The listing builds one solid part. Answer for the finished solid, in the listing's coordinates (mm). Coordinates: 2 decimals unless noted, no trailing zeros. Loops run counter-clockwise (first coordinate to the right, second up) from the corner with the lowest first, then second, coordinate; pieces in that order, holes last. Notation, with made-up numbers: (62.25, 19.25) - (69.25, 19.25) arc R31 cw to (69.25, 47.25) - close; hole circle Ø9 at (3.25, -14.5). An arc over 180 degrees is marked (long way). Put each result on its own line as item: value.
Autodesk Inventor part; units mm, degrees
ref_plane "YZ Plane" through (0, 0, 0) normal (1, 0, 0) x (0, 1, 0)
ref_plane "XZ Plane" through (0, 0, 0) normal (0, 1, 0) x (-1, 0, 0)
ref_plane "XY Plane" through (0, 0, 0) normal (0, 0, 1) x (1, 0, 0)
sketch "Эскиз1" plane through (0, 0, 0) normal (0, 0, 1) x (1, 0, 0)
  arc A0 (68.75, 375.75) -> (58.75, 375.75) centre (63.75, 375.75) ccw
  arc A1 (53.75, 266.5202) -> (58.75, 271.5202) centre (53.75, 271.5202) ccw
  arc A2 (58.75, 246.5202) -> (53.75, 251.5202) centre (53.75, 246.5202) ccw
  arc A3 (-312.25, 375.75) -> (-322.25, 375.75) centre (-317.25, 375.75) ccw
  arc A4 (-312.25, 271.5202) -> (-307.25, 266.5202) centre (-307.25, 271.5202) ccw
  arc A5 (-307.25, 251.5202) -> (-312.25, 246.5202) centre (-307.25, 246.5202) ccw
  arc A6 (-322.25, -155.2817) -> (-312.25, -155.2817) centre (-317.25, -155.2817) ccw
  arc A7 (58.75, -155.2817) -> (68.75, -155.2817) centre (63.75, -155.2817) ccw
  line L0 (68.75, -155.2817) -> (68.75, 375.75)
  line L1 (58.75, 375.75) -> (58.75, 271.5202)
  line L2 (53.75, 266.5202) -> (-307.25, 266.5202)
  line L3 (-307.25, 251.5202) -> (53.75, 251.5202)
  line L4 (58.75, 246.5202) -> (58.75, -155.2817)
  line L5 (-312.25, -155.2817) -> (-312.25, 246.5202)
  line L6 (-312.25, 271.5202) -> (-312.25, 375.75)
  line L7 (-322.25, 375.75) -> (-322.25, -155.2817)
  line L8 (-307.25, 267.0202) -> (53.75, 267.0202)
  arc A8 (53.75, 267.0202) -> (58.25, 271.5202) centre (53.75, 271.5202) ccw
  line L9 (58.25, 271.5202) -> (58.25, 375.75)
  arc A9 (69.25, 375.75) -> (58.25, 375.75) centre (63.75, 375.75) ccw
  line L10 (69.25, 375.75) -> (69.25, -155.2817)
  arc A10 (58.25, -155.2817) -> (69.25, -155.2817) centre (63.75, -155.2817) ccw
  line L11 (58.25, -155.2817) -> (58.25, 246.5202)
  arc A11 (58.25, 246.5202) -> (53.75, 251.0202) centre (53.75, 246.5202) ccw
  line L12 (53.75, 251.0202) -> (-307.25, 251.0202)
  arc A12 (-307.25, 251.0202) -> (-311.75, 246.5202) centre (-307.25, 246.5202) ccw
  line L13 (-311.75, 246.5202) -> (-311.75, -155.2817)
  arc A13 (-322.75, -155.2817) -> (-311.75, -155.2817) centre (-317.25, -155.2817) ccw
  line L14 (-322.75, -155.2817) -> (-322.75, 375.75)
  arc A14 (-311.75, 375.75) -> (-322.75, 375.75) centre (-317.25, 375.75) ccw
  line L15 (-311.75, 375.75) -> (-311.75, 271.5202)
  arc A15 (-311.75, 271.5202) -> (-307.25, 267.0202) centre (-307.25, 271.5202) ccw
  line L16 (-307.25, 266.0202) -> (53.75, 266.0202)
  arc A16 (53.75, 266.0202) -> (59.25, 271.5202) centre (53.75, 271.5202) ccw
  line L17 (59.25, 271.5202) -> (59.25, 375.75)
  arc A17 (68.25, 375.75) -> (59.25, 375.75) centre (63.75, 375.75) ccw
  line L18 (68.25, 375.75) -> (68.25, -155.2817)
  arc A18 (59.25, -155.2817) -> (68.25, -155.2817) centre (63.75, -155.2817) ccw
  line L19 (59.25, -155.2817) -> (59.25, 246.5202)
  arc A19 (59.25, 246.5202) -> (53.75, 252.0202) centre (53.75, 246.5202) ccw
  line L20 (53.75, 252.0202) -> (-307.25, 252.0202)
  arc A20 (-307.25, 252.0202) -> (-312.75, 246.5202) centre (-307.25, 246.5202) ccw
  line L21 (-312.75, 246.5202) -> (-312.75, -155.2817)
  arc A21 (-321.75, -155.2817) -> (-312.75, -155.2817) centre (-317.25, -155.2817) ccw
  line L22 (-321.75, -155.2817) -> (-321.75, 375.75)
  arc A22 (-312.75, 375.75) -> (-321.75, 375.75) centre (-317.25, 375.75) ccw
  line L23 (-312.75, 375.75) -> (-312.75, 271.5202)
  arc A23 (-312.75, 271.5202) -> (-307.25, 266.0202) centre (-307.25, 271.5202) ccw
  point P0 (70, 190)
  dimension "d0" = 0.5
  dimension "d1" = 0.5
extrude "Выдавливание1" add sketch "Эскиз1" along normal blind 7 contours L0 A7 L4 A2 L3 A5 L5 A6 L7 A3 L6 A4 L2 A1 L1 A0 | L8 A8 L9 A9 L10 A10 L11 A11 L12 A12 L13 A13 L14 A14 L15 A15
properties part number "gt2_belt"
1) Each of these flat-tipped pins is pushed along its axis until it touches: pin 1 (2 mm diameter, centred on x = -132, z = 3.5, fed in from +Y); pin 2 (4 mm diameter, centred on x = -245, z = 4, fed in from -Y). Where does it stop, or does it pass through?
Found:
pin 1: stops at y = 267.02
pin 2: stops at y = 251.02
2) The part is cut by section A-A (x = -184.5). Give the vertices of the cut face in (y, z).
Found:
outline: (251.02, 0) - (252.02, 0) - (252.02, 7) - (251.02, 7) - close; (266.02, 0) - (267.02, 0) - (267.02, 7) - (266.02, 7) - close
3) Straight lines are drawn through the part: L1, parallel to X at y = 44, z = 5.5; L2, parallel to Y at x = -80, z = 6.5; L3, parallel to X at y = 253.5, z = 4. For each, find the intervals that lie inside material, in ascending order. Write a range as [from, to].
Found:
L1: x = [-322.75, -321.75], [-312.75, -311.75], [58.25, 59.25], [68.25, 69.25]
L2: y = [251.02, 252.02], [266.02, 267.02]
L3: x = [-322.75, -321.75], [68.25, 69.25]
4) The part is cut by section C-C (y = 334). Give the vertices of the cut face in (x, z), and give its area (3 significant figures).
Found:
outline: (-322.75, 0) - (-321.75, 0) - (-321.75, 7) - (-322.75, 7) - close; (-312.75, 0) - (-311.75, 0) - (-311.75, 7) - (-312.75, 7) - close; (58.25, 0) - (59.25, 0) - (59.25, 7) - (58.25, 7) - close; (68.25, 0) - (69.25, 0) - (69.25, 7) - (68.25, 7) - close
area: 28.0 mm^2
